from build123d import *

# Parameters (mm, degrees)
BOSS_EXTRUDE1_DEPTH             = 5.588
F_1_4_CLEARANCE_HOLE1_D         = 6.35
F_1_4_CLEARANCE_HOLE1_DEPTH     = 5.588
CUT_EXTRUDE1_DEPTH              = 5.588
CUT_EXTRUDE2_REACH              = 7.588
F_4_CLEARANCE_HOLE1_D           = 3.937
F_4_CLEARANCE_HOLE1_DEPTH       = 5.588
CUT_EXTRUDE3_DEPTH              = 5.588
FILLET1_R                       = 0.635
FILLET1_OF_MIRROR2_R            = 0.635
F_10_CLEARANCE_HOLE1_D          = 6.7818
F_10_CLEARANCE_HOLE1_DEPTH      = 5.588
TAP_DRILL_FOR_4_HELICOIL1_D     = 4.064
TAP_DRILL_FOR_4_HELICOIL1_DEPTH = 6.35
TAP_DRILL_FOR_4_HELICOIL1_TIP   = 1.220948778


with BuildPart() as part:
    # Sketch1 → Boss-Extrude1 (new body)
    with BuildSketch(Plane(origin=(0, 0, 0), x_dir=(1, 0, 0), z_dir=(0, 1, 0))):
        with BuildLine():
            Line((-101.6, 50.8), (101.6, 50.8))
            Line((101.6, 50.8), (101.6, 7.9375))
            Line((101.6, 7.9375), (89.172371939, 7.9375))
            ThreePointArc((89.172371939, 7.9375), (87.957352042, 7.695817516), (86.927307909, 7.00756403))
            Line((86.927307909, 7.00756403), (82.164807909, 2.24506403))
            ThreePointArc((82.164807909, 2.24506403), (81.234871939, 0), (82.164807909, -2.24506403))
            Line((82.164807909, -2.24506403), (86.927307909, -7.00756403))
            ThreePointArc((86.927307909, -7.00756403), (87.957352042, -7.695817516), (89.172371939, -7.9375))
            Line((89.172371939, -7.9375), (101.6, -7.9375))
            Line((101.6, -7.9375), (101.6, -50.8))
            Line((101.6, -50.8), (-101.6, -50.8))
            Line((-101.6, -50.8), (-101.6, 50.8))
        make_face()
    extrude(amount=BOSS_EXTRUDE1_DEPTH)

    # 1/4 Clearance Hole1
    with Locations(Plane(origin=(0, 5.588, 0), x_dir=(-1, 0, 0), z_dir=(0, 1, 0))):
        with Locations((-88.10625, 38.1), (-88.10625, -38.1), (88.9, 25.4)):
            Hole(F_1_4_CLEARANCE_HOLE1_D / 2, depth=F_1_4_CLEARANCE_HOLE1_DEPTH)

    # Sketch4 → Cut-Extrude1 (cut)
    with BuildSketch(Plane(origin=(0, 5.588, 0), x_dir=(1, 0, 0), z_dir=(0, 1, 0))):
        with BuildLine():
            Line((88.10625, 41.275), (101.6, 41.275))
            Line((101.6, 41.275), (101.6, 34.925))
            Line((101.6, 34.925), (88.10625, 34.925))
            ThreePointArc((88.10625, 34.925), (84.93125, 38.1), (88.10625, 41.275))
        make_face()
    cut_extrude1 = extrude(amount=-CUT_EXTRUDE1_DEPTH, mode=Mode.SUBTRACT)

    # Mirror1: Cut-Extrude1 across plane
    add(cut_extrude1.mirror(Plane.XY), mode=Mode.SUBTRACT)

    # Sketch5 → Cut-Extrude2 (cut, up to next)
    with BuildSketch(Plane(origin=(0, 5.588, 0), x_dir=(1, 0, 0), z_dir=(0, 1, 0)), mode=Mode.PRIVATE) as cut_extrude2_sk1:
        with BuildLine():
            Line((-92.075, -22.225), (-88.9, -22.225))
            ThreePointArc((-88.9, -22.225), (-85.725, -25.4), (-88.9, -28.575))
            Line((-88.9, -28.575), (-92.075, -28.575))
            ThreePointArc((-92.075, -28.575), (-95.25, -25.4), (-92.075, -22.225))
        make_face()
    cut_extrude2_tool1 = extrude(cut_extrude2_sk1.sketch, amount=-CUT_EXTRUDE2_REACH, mode=Mode.PRIVATE) & part.part
    add(cut_extrude2_tool1.solids().sort_by_distance((-90.4875, 5.588, 25.4))[0], mode=Mode.SUBTRACT)

    # #4 Clearance Hole1
    with Locations(Plane(origin=(0, 5.588, 0), x_dir=(-1, 0, 0), z_dir=(0, 1, 0))):
        with Locations((86.36, -43.18), (35.56, -27.94), (35.56, 0), (87.63, 5.08)):
            Hole(F_4_CLEARANCE_HOLE1_D / 2, depth=F_4_CLEARANCE_HOLE1_DEPTH)

    # Sketch9 → Cut-Extrude3 (cut)
    with BuildSketch(Plane(origin=(0, 5.588, 0), x_dir=(1, 0, 0), z_dir=(0, 1, 0))):
        with BuildLine():
            Line((-6.0325, 18.7198), (6.0325, 18.7198))
            ThreePointArc((6.0325, 18.7198), (6.574506403, 18.944306403), (6.35, 18.4023))
            Line((6.35, 18.4023), (6.35, 13.0175))
            ThreePointArc((6.35, 13.0175), (6.574506403, 12.475493597), (6.0325, 12.7))
            Line((6.0325, 12.7), (-6.0325, 12.7))
            ThreePointArc((-6.0325, 12.7), (-6.574506403, 12.475493597), (-6.35, 13.0175))
            Line((-6.35, 13.0175), (-6.35, 18.4023))
            ThreePointArc((-6.35, 18.4023), (-6.574506403, 18.944306403), (-6.0325, 18.7198))
        make_face()
        with BuildLine():
            Line((57.15, 18.4023), (57.15, 13.0175))
            ThreePointArc((57.15, 13.0175), (56.925493597, 12.475493597), (57.4675, 12.7))
            Line((57.4675, 12.7), (69.5325, 12.7))
            ThreePointArc((69.5325, 12.7), (70.074506403, 12.475493597), (69.85, 13.0175))
            Line((69.85, 13.0175), (69.85, 18.4023))
            ThreePointArc((69.85, 18.4023), (70.074506403, 18.944306403), (69.5325, 18.7198))
            Line((69.5325, 18.7198), (57.4675, 18.7198))
            ThreePointArc((57.4675, 18.7198), (56.925493597, 18.944306403), (57.15, 18.4023))
        make_face()
    cut_extrude3 = extrude(amount=-CUT_EXTRUDE3_DEPTH, mode=Mode.SUBTRACT)

    # Fillet1
    fillet1_edges = [part.edges().sort_by_distance(p)[0] for p in [
        (-6.35, 2.794, -18.4023),
        (-6.0325, 2.794, -18.7198),
        (6.0325, 2.794, -18.7198),
        (6.35, 2.794, -18.4023),
        (6.35, 2.794, -13.0175),
        (6.0325, 2.794, -12.7),
        (-6.0325, 2.794, -12.7),
        (-6.35, 2.794, -13.0175),
        (69.85, 2.794, -13.0175),
        (69.5325, 2.794, -12.7),
        (57.4675, 2.794, -12.7),
        (57.15, 2.794, -13.0175),
        (57.15, 2.794, -18.4023),
        (57.4675, 2.794, -18.7198),
        (69.5325, 2.794, -18.7198),
        (69.85, 2.794, -18.4023),
    ]]
    fillet(fillet1_edges, radius=FILLET1_R)

    # Mirror2: Cut-Extrude3 across plane
    add(cut_extrude3.mirror(Plane.XY), mode=Mode.SUBTRACT)

    # Fillet1 of Mirror2
    fillet1_of_mirror2_edges = [part.edges().sort_by_distance(p)[0] for p in [
        (-6.35, 2.794, 18.4023),
        (-6.0325, 2.794, 18.7198),
        (6.0325, 2.794, 18.7198),
        (6.35, 2.794, 18.4023),
        (6.35, 2.794, 13.0175),
        (6.0325, 2.794, 12.7),
        (-6.0325, 2.794, 12.7),
        (-6.35, 2.794, 13.0175),
        (69.85, 2.794, 13.0175),
        (69.5325, 2.794, 12.7),
        (57.4675, 2.794, 12.7),
        (57.15, 2.794, 13.0175),
        (57.15, 2.794, 18.4023),
        (57.4675, 2.794, 18.7198),
        (69.5325, 2.794, 18.7198),
        (69.85, 2.794, 18.4023),
    ]]
    fillet(fillet1_of_mirror2_edges, radius=FILLET1_OF_MIRROR2_R)

    # #10 Clearance Hole1
    with Locations(Plane(origin=(0, 5.588, 0), x_dir=(-1, 0, 0), z_dir=(0, 1, 0))):
        with Locations((-19.05, 0), (-44.45, 0)):
            Hole(F_10_CLEARANCE_HOLE1_D / 2, depth=F_10_CLEARANCE_HOLE1_DEPTH)

    # Tap Drill for #4 Helicoil1
    with Locations(Plane(origin=(0, 5.588, 0), x_dir=(1, 0, 0), z_dir=(0, 1, 0))):
        with Locations((93.4847, 18.7325), (83.9597, 18.7325)):
            Hole(TAP_DRILL_FOR_4_HELICOIL1_D / 2, depth=TAP_DRILL_FOR_4_HELICOIL1_DEPTH)
            with Locations((0, 0, -(TAP_DRILL_FOR_4_HELICOIL1_DEPTH + TAP_DRILL_FOR_4_HELICOIL1_TIP / 2))):  # 118° drill point
                Cone(0, TAP_DRILL_FOR_4_HELICOIL1_D / 2, TAP_DRILL_FOR_4_HELICOIL1_TIP, mode=Mode.SUBTRACT)


solid = part.part
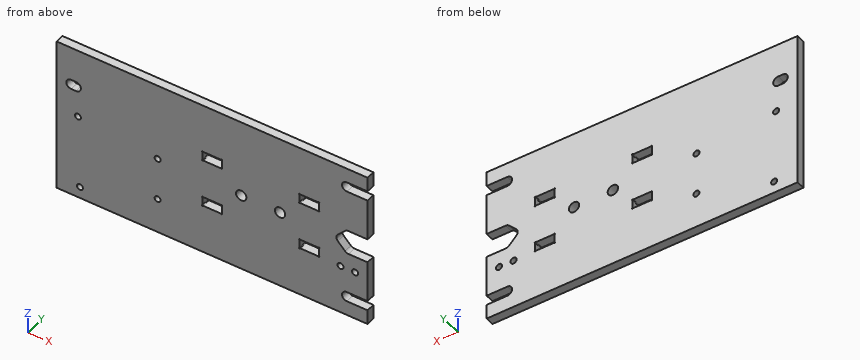
The listing builds one solid part. Answer for the finished solid, in the listing's coordinates (mm). Give positions to 0.01 mm unless a question says otherwise; leave off trailing zeros. Loops run counter-clockwise (first coordinate to the right, second up) from the corner with the lowest first, then second, coordinate; pieces in that order, holes last. Notation, with made-up numbers: M -7,-10 L 15,-10 A16 ccw 15,0 Z; hole C 24,89 d6. An arc over 180 degrees is marked long. Answer as CSV lines item,"result".
Item 1: The part is cut by section A-A (z = 0). Give the vertices of the cut face in (x, y), and give its area (3 significant figures).
Values follow:
outline,"M -101.6,0 L -37.53,0 L -37.53,5.59 L -101.6,5.59 Z; M -33.59,0 L 15.66,0 L 15.66,5.59 L -33.59,5.59 Z; M 22.44,0 L 41.06,0 L 41.06,5.59 L 22.44,5.59 Z; M 47.84,0 L 81.23,0 L 81.23,5.59 L 47.84,5.59 Z"
area,"924 mm^2"
Item 2: Given pin 1 Ø3 at (x, z) = (78, -32) entering from -Y, flat-ended and moving along its own axis, determine where the tip first touches the part or whether it passes through.
Values follow:
pin 1,"stops at y = 0"
Item 3: Straight lines are drawn through the part: line 1 along Z through (x, y) = (19.05, 2); line 2 along X through (y, z) = (4.15, 38); line 3 along Z through (x, y) = (45, 0.85). For each, find the intervals that lie inside material, in ascending order. Write a range as [from, to].
Values follow:
line 1,"z = [-50.8, -3.39], [3.39, 50.8]"
line 2,"x = [-101.6, 84.93]"
line 3,"z = [-50.8, -3.35], [3.35, 50.8]"
Item 4: The part is cut by section D-D (y = 3.2). Give the number of separate pieces and of enclosed holes in the cut face, and give its area (3 significant figures).
Values follow:
separate pieces,"1"
enclosed holes,"13"
area,"19,700 mm^2"
Item 5: The part is cut by section C-C (z = 38.1). Give the vertices of the cut face in (x, y), and give its area (3 significant figures).
Values follow:
outline,"M -101.6,0 L 84.93,0 L 84.93,5.59 L -101.6,5.59 Z"
area,"1,040 mm^2"
Item 6: The part is cut by section B-B (x = 44.45). Give the vertices of the cut face in (y, z), and give its area (3 significant figures).
Values follow:
outline,"M 0,-50.8 L 5.59,-50.8 L 5.59,-3.39 L 0,-3.39 Z; M 0,3.39 L 5.59,3.39 L 5.59,50.8 L 0,50.8 Z"
area,"530 mm^2"
